Verification items for the finished model (mm, model axes). A direction names the side the tool comes from. Round coordinates to 2 decimals unless told otherwise and drop trailing zeros. Write each loop counter-clockwise with the first axis right and the second up, starting at its lowest first coordinate (ties: lowest second). Pieces come first, ordered by that corner, then holes. Notation, with made-up numbers: M -29.75,36.25 L -19.75,36.25 A28 cw -19.75,58.25 Z; hole C 88.5,-24 d2. An arc over 180 degrees is marked long. One line per question, with ' | ' between items.
from build123d import *

# Parameters (mm, degrees)
F0_W     = 900
F0_H     = 2000
F0_W_2   = 800
F0_H_2   = 300
F0_H_3   = 350
F1_DEPTH = 500


with BuildPart() as f1:
    # F0 (on Front) → F1 (new body)
    with BuildSketch(Plane.XZ):
        Rectangle(F0_W, F0_H)
        with Locations((0, -800)):
            Rectangle(F0_W_2, F0_H_2, mode=Mode.SUBTRACT)
        with Locations((0, -425)):
            Rectangle(F0_W_2, F0_H_3, mode=Mode.SUBTRACT)
        with Locations((0, -25)):
            Rectangle(F0_W_2, F0_H_3, mode=Mode.SUBTRACT)
        with Locations((0, 375)):
            Rectangle(F0_W_2, F0_H_3, mode=Mode.SUBTRACT)
        with Locations((0, 775)):
            Rectangle(F0_W_2, F0_H_3, mode=Mode.SUBTRACT)
    extrude(amount=F1_DEPTH)


solid = f1.part
1. Section check B-B, the plane z = -370.5. Record the cut outline in (x, y).
Results:
outline: M -450,-500 L -400,-500 L -400,0 L -450,0 Z; M 400,-500 L 450,-500 L 450,0 L 400,0 Z
2. Section check C-C, the plane y = -77. Record the cut outline in (x, z), then the cut area to 3 significant figures.
Results:
outline: M -450,-1000 L 450,-1000 L 450,1000 L -450,1000 Z; hole M -400,-950 L 400,-950 L 400,-650 L -400,-650 Z; hole M -400,-600 L 400,-600 L 400,-250 L -400,-250 Z; hole M -400,-200 L 400,-200 L 400,150 L -400,150 Z; hole M -400,200 L 400,200 L 400,550 L -400,550 Z; hole M -400,600 L 400,600 L 400,950 L -400,950 Z | area: 440,000 mm2
3. Tool access check on faces 1 (the face through (-6, -246, -1000)), 2 (the face through (-6, -246, -200)). Record the directions out of +Z, -Z, +X, -X, +Y, -Y that give a thin tool (end or side, any length) a straight path to the whole face; none if there is none.
Results:
face 1: -Z, +X, -X, +Y, -Y | face 2: +Y, -Y
4. Section check A-A, the plane x = 57. Record the cut outline in (y, z), then the cut area to 3 significant figures.
Results:
outline: M -500,-1000 L 0,-1000 L 0,-950 L -500,-950 Z; M -500,-650 L 0,-650 L 0,-600 L -500,-600 Z; M -500,-250 L 0,-250 L 0,-200 L -500,-200 Z; M -500,150 L 0,150 L 0,200 L -500,200 Z; M -500,550 L 0,550 L 0,600 L -500,600 Z; M -500,950 L 0,950 L 0,1000 L -500,1000 Z | area: 150,000 mm2
5. Thickness scan on line 1 (Z direction, x = 188, y = -392); line 2 (X direction, y = -69.5, z = -367.5). Record the ranges inside material, lowest first.
Results:
line 1: z = -1000 to -950, -650 to -600, -250 to -200, 150 to 200, 550 to 600, 950 to 1000 | line 2: x = -450 to -400, 400 to 450
6. Mould release check, pull along X, two halves, no side actions. Record for faces 3 (the face through (-69, 0, 153)), 4 (the face through (450, -246, -14)), 5 (the face through (400, -246, -427)): pulls with the +X half, pulls with the -X half, needs draft (parallel to the pull), parting line crosses it, or undercut.
Results:
face 3: needs draft | face 4: pulls with the +X half | face 5: undercut
